from build123d import *

# Parameters (mm, degrees)
SKETCH_1_W          = 20
SKETCH_1_H          = 20
EXTRUDE_1_DEPTH     = 80
SKETCH_3_W          = 30
SKETCH_3_H          = 20
EXTRUDE_2_DEPTH     = 5
SKETCH_4_R          = 2.9
CUT_EXTRUDE_1_DEPTH = 10


with BuildPart() as part:
    # 草图1 → 凸台-拉伸1 (new body)
    with BuildSketch(Plane(origin=(0, 0, 0), x_dir=(1, 0, 0), z_dir=(0, 1, 0))):
        Rectangle(SKETCH_1_W, SKETCH_1_H)
    extrude(amount=EXTRUDE_1_DEPTH)

    # 草图3 → 凸台-拉伸2 (add)
    with BuildSketch(Plane(origin=(0, 0, 0), x_dir=(-1, 0, 0), z_dir=(0, -1, 0))):
        with Locations((-5, 0)):
            Rectangle(SKETCH_3_W, SKETCH_3_H)
    extrude(amount=EXTRUDE_2_DEPTH)

    # 草图4 → 切除-拉伸1 (cut)
    with BuildSketch(Plane(origin=(0, 80, 0), x_dir=(1, 0, 0), z_dir=(0, 1, 0))):
        with Locations(Location((0, 0, 0), (0, 0, 270))):
            Circle(SKETCH_4_R)
    extrude(amount=-CUT_EXTRUDE_1_DEPTH, mode=Mode.SUBTRACT)


solid = part.part
The model under review builds one solid part; all positions refer to its coordinate system, in mm. A direction names the side the tool comes from. Coordinates: 2 decimals unless noted, no trailing zeros. Loops run counter-clockwise (first coordinate to the right, second up) from the corner with the lowest first, then second, coordinate; pieces in that order, holes last.
(1) Insertion check: P1, Ø4, axis at y = 67.5, z = 7, coming from the +X side; P2, Ø3, axis at x = 14.5, z = -1.5, coming from the +Y side. Each pin has a flat end and moves straight along its axis. Give the tip position at first contact, or say it passes through.
Determined:
P1: stops at x = 10
P2: stops at y = 0
(2) Draft analysis for pull direction Z (two halves, no side actions). For faces 1 (the flat face through (-10, 38, 0)), 2 (the flat face through (-1, 38, -10)), 3 (the flat face through (0, 70, 0)), state which applies: +Z half, -Z half, draft (parallel to the pull), parting line (faces both ways), or undercut.
Determined:
face 1: draft
face 2: -Z half
face 3: undercut
(3) Wall thickness on L1, parallel to X at y = 73, z = 0; L2, parallel to X at y = 50, z = 6.75; L3, parallel to Y at x = 14.25, z = -0.5: over which ranges is each line inside the solid? List them lowest first.
Determined:
L1: x = -10 to -2.9, 2.9 to 10
L2: x = -10 to 10
L3: y = -5 to 0
(4) Consider section A-A, the plane z = 0. Give the boundary of the cut face in (x, y).
Determined:
outline: (-10, -5) - (20, -5) - (20, 0) - (10, 0) - (10, 80) - (2.9, 80) - (2.9, 70) - (-2.9, 70) - (-2.9, 80) - (-10, 80) - close
(5) Consider section C-C, the plane y = 62. Give the boundary of the cut face in (x, z).
Determined:
outline: (-10, -10) - (10, -10) - (10, 10) - (-10, 10) - close
(6) Tool access review of faces 4 (the flat face through (10, 39, 0)), 5 (the cylindrical face through (0.1, 75.1, -2.9)), 6 (the flat face through (-1, 38, 10)): name each direction out of +Z, -Z, +X, -X, +Y, -Y from which nothing blocks a thin tool from reaching the whole face with its end or side.
Determined:
face 4: +Z, -Z, +X, +Y
face 5: +Y
face 6: +Z, +X, -X, +Y, -Y
(7) Consider section B-B, the plane x = 14.5. Give the boundary of the cut face in (y, z).
Determined:
outline: (-5, -10) - (0, -10) - (0, 10) - (-5, 10) - close
(8) Consider section D-D, the plane z = 5. Give the boundary of the cut face in (x, y), plus the area to 3 significant figures.
Determined:
outline: (-10, -5) - (20, -5) - (20, 0) - (10, 0) - (10, 80) - (-10, 80) - close
area: 1,750 mm2
